For this review, take the finished solid that the model builds, in its own axes (mm). Give positions to 0.01 mm unless a question says otherwise; leave off trailing zeros. Order: outer loops, then holes, each group sorted by start corner. A loop starts at its lowest first (then second) coordinate and runs counter-clockwise, first axis right, second up. Notation, with made-up numbers: (-24.75, -25.75) - (33.25, -25.75) arc R21 cw to (33.25, -6.75) - close; hole circle Ø7 at (78.25, 60). An arc over 180 degrees is marked (long way). One line per item, written item: value.
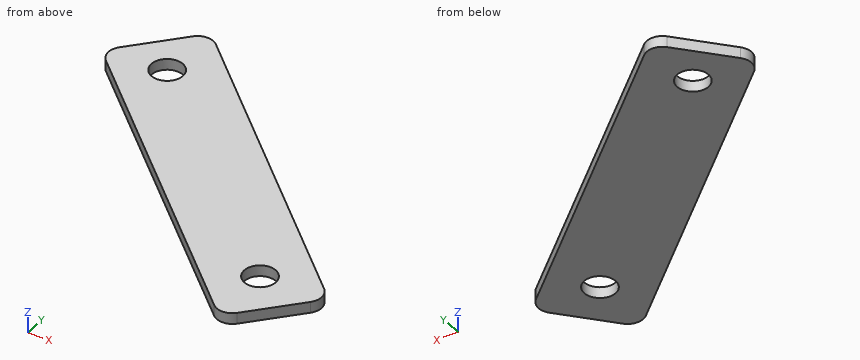
```python
from build123d import *

# Parameters (mm, degrees)
BOSS_EXTRUDE1_DEPTH = 7
FILLET1_R           = 10
SKETCH3_R           = 10
CUT_EXTRUDE1_DEPTH  = 7
SCALE1_SCALE        = 0.2
SCALE2_SCALE        = 2.5
SCALE3_SCALE        = 0.8


with BuildPart() as part:
    # Sketch1 → Boss-Extrude1 (new body)
    with BuildSketch(Plane.XY):
        Polygon((0, 0), (40.058778279, 44.668717049), (-146.060876092, 211.580293211), (-186.119654371, 166.911576162), align=None)
    extrude(amount=BOSS_EXTRUDE1_DEPTH)

    # Fillet1
    fillet1_edges = [part.edges().sort_by_distance(p)[0] for p in [
        (-186.119654371, 166.911576162, 3.5),
        (-146.060876092, 211.580293211, 3.5),
        (40.058778279, 44.668717049, 3.5),
        (0, 0, 3.5),
    ]]
    fillet(fillet1_edges, radius=FILLET1_R)

    # Sketch3 → Cut-Extrude1 (cut)
    with BuildSketch(Plane.XY.offset(7)):
        with Locations((-1.778551095, 41.89165724)):
            Circle(SKETCH3_R)
        with Locations((-147.041782503, 171.152655791)):
            Circle(SKETCH3_R)
    extrude(amount=-CUT_EXTRUDE1_DEPTH, mode=Mode.SUBTRACT)


with BuildPart() as part_1:
    # Scale1: scaled about (-72.969754943, 105.757951413, 3.5)
    add(part.part.scale(SCALE1_SCALE).moved(Location((-58.375803954, 84.60636113, 2.8))))


with BuildPart() as part_2:
    # Scale2: scaled about (-72.969754943, 105.757951413, 3.5)
    add(part_1.part.scale(SCALE2_SCALE).moved(Location((109.454632414, -158.63692712, -5.25))))


with BuildPart() as part_3:
    # Scale3: scaled about (-72.969754943, 105.757951413, 3.5)
    add(part_2.part.scale(SCALE3_SCALE).moved(Location((-14.593950989, 21.151590283, 0.7))))


solid = part_3.part
```
(1) Take a section at A-A (z = 3.9). Write out the cut boundary in (x, y).
Answers below:
outline: (-115.56, 133.2) arc R4 ccw to (-115.25, 127.55) - (-46.76, 66.13) arc R4 ccw to (-41.11, 66.43) - (-30.43, 78.34) arc R4 ccw to (-30.74, 83.99) - (-99.23, 145.42) arc R4 ccw to (-104.88, 145.11) - close; hole circle Ø8 at (-102.6, 131.92); hole circle Ø8 at (-44.49, 80.21)
(2) Wall thickness on line 1 (Y direction, x = -102, z = 2.5); line 2 (Y direction, x = -47.5, z = 4.65); line 3 (Y direction, x = -68.5, z = 4.2): over which ranges is each line inside the solid? List them lowest first. Write a range as from..to.
Answers below:
line 1: y = 115.66..127.96, 135.87..146.44
line 2: y = 66.79..77.57, 82.85..99.03
line 3: y = 85.62..117.86
(3) Take a section at C-C (y = 99.5). Write out the cut boundary in (x, z), then the cut area to 3 significant figures.
Answers below:
outline: (-83.98, 2.1) - (-48.03, 2.1) - (-48.03, 4.9) - (-83.98, 4.9) - close
area: 101 mm^2
(4) Take a section at B-B (x = -103.5). Write out the cut boundary in (y, z).
Answers below:
outline: (117.01, 2.1) - (128.02, 2.1) - (128.02, 4.9) - (117.01, 4.9) - close; (135.81, 2.1) - (146.1, 2.1) - (146.1, 4.9) - (135.81, 4.9) - close
(5) For P1, Ø1, axis at y = 123.5, z = 3.5, coming from the -X side, flat-tipped, find the tip position at first contact; note if it passes through.
Answers below:
P1: stops at x = -111.29
(6) Take a section at D-D (x = -63.5). Write out the cut boundary in (y, z).
Answers below:
outline: (81.14, 2.1) - (113.38, 2.1) - (113.38, 4.9) - (81.14, 4.9) - close
